from build123d import *

# Parameters (mm, degrees)
SKETCH1_R           = 16.75
BOSS_EXTRUDE1_DEPTH = 15
SHELL2_T            = -0.5
FILLET1_R           = 0.5


with BuildPart() as part:
    # Sketch1 → Boss-Extrude1 (new body)
    with BuildSketch(Plane.XY):
        Circle(SKETCH1_R)
    extrude(amount=BOSS_EXTRUDE1_DEPTH)

    # Shell2
    shell2_openings = [part.faces().sort_by_distance(p)[0] for p in [
        (0, 0, 15),
    ]]
    offset(amount=SHELL2_T, openings=shell2_openings, kind=Kind.INTERSECTION)

    # Fillet1
    fillet1_edges = [part.edges().sort_by_distance(p)[0] for p in [
        (-16.75, 0, 0),
    ]]
    fillet(fillet1_edges, radius=FILLET1_R)


solid = part.part
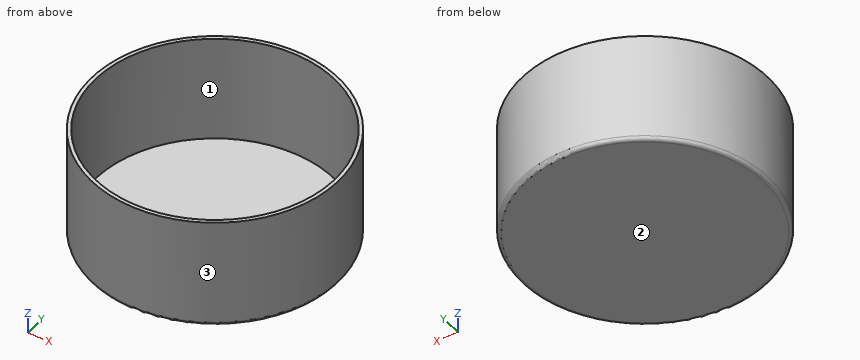
Model file for the job. Use its own axes, mm. Face numbers are marked on the shaded views. Give positions to 0.01 mm unless a question says otherwise; leave off trailing zeros. Order: outer loops, then holes, each group sorted by start corner. A loop starts at its lowest first (then second) coordinate and runs counter-clockwise, first axis right, second up. Notation, with made-up numbers: M 46,79 L 97,79 A26 cw 97,117 Z; hole C 50.5,1.5 d9. An arc over 180 degrees is marked long. Write item = value, one per line.
Q1. Drill centre lines: line 1 (Y direction, x = 0.5, z = 10.5); line 2 (Z direction, x = 5.5, y = 14.5); line 3 (Y direction, x = 3.5, z = 6.75). Where is each one in solid material? Low to high. Write a range as [from, to].
Derived:
line_1 = [-16.74, -16.24], [16.24, 16.74]
line_2 = [0, 0.5]
line_3 = [-16.38, -15.87], [15.87, 16.38]
Q2. Cut at A-A, the plane x = 0. List the corners of the cut face in (y, z), then the cut area to 3 significant figures.
Derived:
outline = M -16.75,0.5 A0.5 ccw -16.25,0 L 16.25,0 A0.5 ccw 16.75,0.5 L 16.75,15 L 16.25,15 L 16.25,0.5 L -16.25,0.5 L -16.25,15 L -16.75,15 Z
area = 31.1 mm2
Q3. Two-plate mould, pull along Y, no slides. Class the marked faces 1, 2 and 3: pulls with the +Y half, pulls with the -Y half, needs draft (parallel to the pull), parting line crosses it, or undercut.
Derived:
face_1 = undercut
face_2 = needs draft
face_3 = parting line crosses it
Q4. Cut at B-B, the plane z = 12.75. List the corners of the cut face in (x, y).
Derived:
outline = C 0,0 d33.5; hole C 0,0 d32.5
Q5. Flat gauge pins, fed straight in: pin 1 (1.5 mm diameter, centred on x = -11, z = 7.5, fed in from -Y); pin 2 (16 mm diameter, centred on x = -1, y = -3, fed in from +Z); pin 3 (4 mm diameter, centred on y = 7.5, z = 5, fed in from -X). Where does each tip first touch, or does it go through?
Derived:
pin_1 = -13.25
pin_2 = 0.5
pin_3 = -15.82
